```python
from build123d import *

# Parameters (mm, degrees)
SKETCH_R        = 2.1
SKETCH_R_2      = 11
SKETCH_R_3      = 20
SKETCH_R_4      = 1.65
PAD_DEPTH       = 10
SKETCH001_R     = 23.5
POCKET_DEPTH    = 7
SKETCH002_R     = 14
POCKET001_DEPTH = 3


with BuildPart() as part:
    # Sketch → Pad (new body)
    with BuildSketch(Plane.XY):
        with BuildLine():
            ThreePointArc((0, 60), (-60, 0), (0, -60))
            Line((155, -60), (0, -60))
            Line((155, 60), (155, -60))
            Line((0, 60), (155, 60))
        make_face()
        with Locations((84.5, -54.5)):
            Circle(SKETCH_R, mode=Mode.SUBTRACT)
        with Locations((84.5, 54.5)):
            Circle(SKETCH_R, mode=Mode.SUBTRACT)
        with Locations((149.5, 54.5)):
            Circle(SKETCH_R, mode=Mode.SUBTRACT)
        with Locations((149.5, -54.5)):
            Circle(SKETCH_R, mode=Mode.SUBTRACT)
        with Locations((-45.5, 30)):
            Circle(SKETCH_R, mode=Mode.SUBTRACT)
        with Locations((-45.5, -30)):
            Circle(SKETCH_R, mode=Mode.SUBTRACT)
        with Locations((19.5, 54.5)):
            Circle(SKETCH_R, mode=Mode.SUBTRACT)
        with Locations((19.5, -54.5)):
            Circle(SKETCH_R, mode=Mode.SUBTRACT)
        with Locations((106.5, -27)):
            Circle(SKETCH_R, mode=Mode.SUBTRACT)
        with Locations((137.5, -27)):
            Circle(SKETCH_R, mode=Mode.SUBTRACT)
        with Locations((149.5, 30)):
            Circle(SKETCH_R, mode=Mode.SUBTRACT)
        with Locations((106.5, 27)):
            Circle(SKETCH_R, mode=Mode.SUBTRACT)
        with Locations((79, 0)):
            Circle(SKETCH_R_2, mode=Mode.SUBTRACT)
        Circle(SKETCH_R_3, mode=Mode.SUBTRACT)
        with Locations((-28.284271, 28.284271)):
            Circle(SKETCH_R, mode=Mode.SUBTRACT)
        with Locations((28.284271, 28.284271)):
            Circle(SKETCH_R, mode=Mode.SUBTRACT)
        with Locations((-28.284271, -28.284271)):
            Circle(SKETCH_R, mode=Mode.SUBTRACT)
        with Locations((28.284271, -28.284271)):
            Circle(SKETCH_R, mode=Mode.SUBTRACT)
        with Locations((79, -16)):
            Circle(SKETCH_R, mode=Mode.SUBTRACT)
        with Locations((92.856406, 8)):
            Circle(SKETCH_R, mode=Mode.SUBTRACT)
        with Locations((65.143594, 8)):
            Circle(SKETCH_R, mode=Mode.SUBTRACT)
        with Locations((48, 2)):
            Circle(SKETCH_R_4, mode=Mode.SUBTRACT)
        with Locations((56.39, -2.46)):
            Circle(SKETCH_R_4, mode=Mode.SUBTRACT)
        with Locations((149.5, -30)):
            Circle(SKETCH_R, mode=Mode.SUBTRACT)
        with Locations((137.5, 27)):
            Circle(SKETCH_R, mode=Mode.SUBTRACT)
        with BuildLine():
            Line((104.5, 21.5), (147.5, 21.5))
            ThreePointArc((149, 20), (148.56066, 21.06066), (147.5, 21.5))
            Line((149, 20), (149, -20))
            ThreePointArc((147.5, -21.5), (148.56066, -21.06066), (149, -20))
            Line((147.5, -21.5), (104.5, -21.5))
            ThreePointArc((103, -20), (103.43934, -21.06066), (104.5, -21.5))
            Line((103, -20), (103, 20))
            ThreePointArc((104.5, 21.5), (103.43934, 21.06066), (103, 20))
        make_face(mode=Mode.SUBTRACT)
        with BuildLine():
            ThreePointArc((47.5, 24), (45, 26.5), (42.5, 24))
            Line((42.5, 24), (42.5, 12))
            ThreePointArc((42.5, 12), (45, 9.5), (47.5, 12))
            Line((47.5, 24), (47.5, 12))
        make_face(mode=Mode.SUBTRACT)
        with BuildLine():
            ThreePointArc((47.5, -12), (45, -9.5), (42.5, -12))
            Line((42.5, -12), (42.5, -24))
            ThreePointArc((42.5, -24), (45, -26.5), (47.5, -24))
            Line((47.5, -12), (47.5, -24))
        make_face(mode=Mode.SUBTRACT)
    extrude(amount=PAD_DEPTH)

    # Sketch001 (on Face47 of Pad) → Pocket (cut)
    with BuildSketch(Plane.XY.offset(10)):
        Circle(SKETCH001_R)
    extrude(amount=-POCKET_DEPTH, mode=Mode.SUBTRACT)

    # Sketch002 (on Face5 of Pocket) → Pocket001 (cut)
    with BuildSketch(Plane.XY.offset(10)):
        with Locations((79, 0)):
            Circle(SKETCH002_R)
    extrude(amount=-POCKET001_DEPTH, mode=Mode.SUBTRACT)


solid = part.part
```
Geometry check sheet. Reference: the model listing, model coordinates, mm. A direction names the side the tool comes from. Round coordinates to 2 decimals unless told otherwise and drop trailing zeros. Loops run counter-clockwise (first coordinate to the right, second up) from the corner with the lowest first, then second, coordinate; pieces in that order, holes last. Notation, with made-up numbers: (48.5, 51.5) - (98.5, 51.5) arc R36 ccw to (98.5, 90.5) - close; hole circle Ø10 at (-20.75, 58.5). An arc over 180 degrees is marked (long way). Use a Markdown table: item, result.
Q1. Draft check along Y on faces 1 (the cylindrical face through (66.78, -6.83, 8.52)), 2 (the flat face through (76, 60, 5)), 3 (the cylindrical face through (-29.95, -29.56, 4.93)), 4 (the flat face through (46, 1, 10)). Enter one of: released by +Y, released by -Y, zero draft, split by the parting line, or undercut.
Solutions:
| item | result |
|---|---|
| face 1 | undercut |
| face 2 | released by +Y |
| face 3 | undercut |
| face 4 | zero draft |
Q2. Cross-section at C-C on y = 54.5. Record the cut outline in (x, z), plus the area to 3 significant figures.
Solutions:
| item | result |
|---|---|
| outline | (-25.09, 0) - (17.4, 0) - (17.4, 10) - (-25.09, 10) - close; (21.6, 0) - (82.4, 0) - (82.4, 10) - (21.6, 10) - close; (86.6, 0) - (147.4, 0) - (147.4, 10) - (86.6, 10) - close; (151.6, 0) - (155, 0) - (155, 10) - (151.6, 10) - close |
| area | 1,670 mm2 |
Q3. Cross-section at A-A on x = 112. Record the cut outline in (y, z).
Solutions:
| item | result |
|---|---|
| outline | (-60, 0) - (-21.5, 0) - (-21.5, 10) - (-60, 10) - close; (21.5, 0) - (60, 0) - (60, 10) - (21.5, 10) - close |
Q4. Go/stop test with flat-tipped pins: P1, Ø2, axis at y = -16, z = 6.5, coming from the -X side; P2, Ø5.5, axis at x = 28.28, y = -28.28, coming from the -Z side; P3, Ø6, axis at y = -20, z = 5.5, coming from the -X side; P4, Ø3, axis at y = 1.5, z = 7, coming from the -X side. Record where each tip stops, or that it passes through.
Solutions:
| item | result |
|---|---|
| P1 | stops at x = -58.09 |
| P2 | stops at z = 0 |
| P3 | stops at x = -57.54 |
| P4 | stops at x = -60 |
Q5. Material ranges on line 1 (Y direction, x = 106.5, z = 4.25); line 2 (Y direction, x = 79, z = 2.5); line 3 (Y direction, x = 149.5, z = 3.25), recorded low to high.
Solutions:
| item | result |
|---|---|
| line 1 | y = -60 to -29.1, -24.9 to -21.5, 21.5 to 24.9, 29.1 to 60 |
| line 2 | y = -60 to -18.1, -13.9 to -11, 11 to 60 |
| line 3 | y = -60 to -56.6, -52.4 to -32.1, -27.9 to 27.9, 32.1 to 52.4, 56.6 to 60 |
Q6. Cross-section at B-B on y = -16. Record the cut outline in (x, z), plus the area to 3 significant figures.
Solutions:
| item | result |
|---|---|
| outline | (-57.83, 0) - (-12, 0) - (-12, 3) - (-17.21, 3) - (-17.21, 10) - (-57.83, 10) - close; (12, 0) - (42.5, 0) - (42.5, 10) - (17.21, 10) - (17.21, 3) - (12, 3) - close; (47.5, 0) - (76.9, 0) - (76.9, 10) - (47.5, 10) - close; (81.1, 0) - (103, 0) - (103, 10) - (81.1, 10) - close; (149, 0) - (155, 0) - (155, 10) - (149, 10) - close |
| area | 1,260 mm2 |
Q7. Access from +Z, -Z, +X, -X, +Y, -Y to the whole of each face (thin tool, end or side, straight path). Record for faces 5 (the flat face through (7, 19, 3)), 6 (the flat face through (42.5, -18, 5)), 7 (the flat face through (155, 1, 5)).
Solutions:
| item | result |
|---|---|
| face 5 | +Z |
| face 6 | +Z, -Z |
| face 7 | +Z, -Z, +X, +Y, -Y |
Q8. Cross-section at D-D on x = 10. Record the cut outline in (y, z).
Solutions:
| item | result |
|---|---|
| outline | (-60, 0) - (-17.32, 0) - (-17.32, 3) - (-21.27, 3) - (-21.27, 10) - (-60, 10) - close; (17.32, 0) - (60, 0) - (60, 10) - (21.27, 10) - (21.27, 3) - (17.32, 3) - close |
